Drawing for the job (mm, zero at the part's lowest x, y, z). A direction names the side the tool comes from. Give positions to 0.01 mm unless a question says otherwise; leave off trailing zeros. Order: outer loops, then holes, each group sorted by start corner. A loop starts at its lowest first (then second) coordinate and runs counter-clockwise, first axis right, second up. Notation, with made-up numbers: (-6.5, 76) - (31.5, 76) arc R29 cw to (31.5, 104) - close; hole circle Ø4 at (49, 68.25). An arc over 180 degrees is marked (long way). Use CSV: the item, a comma, the result in double quotes. Start each with the question number.
(1) Band-saw the part on B-B, the plane y = 8.75. Give the cut face in (x, z).
(2) Tool access for the marked faces 1, 2 and 3: list every direction of +Z, -Z, +X, -X, +Y, -Y with a clear straight run to the whole face (end or side of a thin tool).
(3) Pull direction X, two halves, no side cores. Call the marked faces 4, 5 and 6: +X half, -X half, draft (parallel to the pull), parting line (faces both ways), or undercut.
(4) Drop flat-ended pins along their axis: pin 1 Ø24 at (x, z) = (36, 52.5) entering from -Y; pin 2 Ø3 at (y, z) = (20.5, 39) entering from +X; pin 3 Ø2 at (x, z) = (44.5, 67) entering from +Y; pin 4 Ø10 at (y, z) = (3.5, 12.5) entering from +X. Give the stop position or say it passes through.
(5) Probe L1, parallel to Z at x = 50, y = 7; L2, parallel to X at y = 8, z = 59; L3, parallel to Z at x = 50, y = 12.75. List the from-to ranges inside material, lowest first.
(6) Band-saw the part on C-C, the plane z = 50. Give the cut face in (x, y).
(7) Band-saw the part on A-A, the plane x = 50. Give the cut face in (y, z), then the cut area to 3 significant figures.
(8) Band-saw the part on D-D, the plane z = 65. Give the cut face in (x, y).
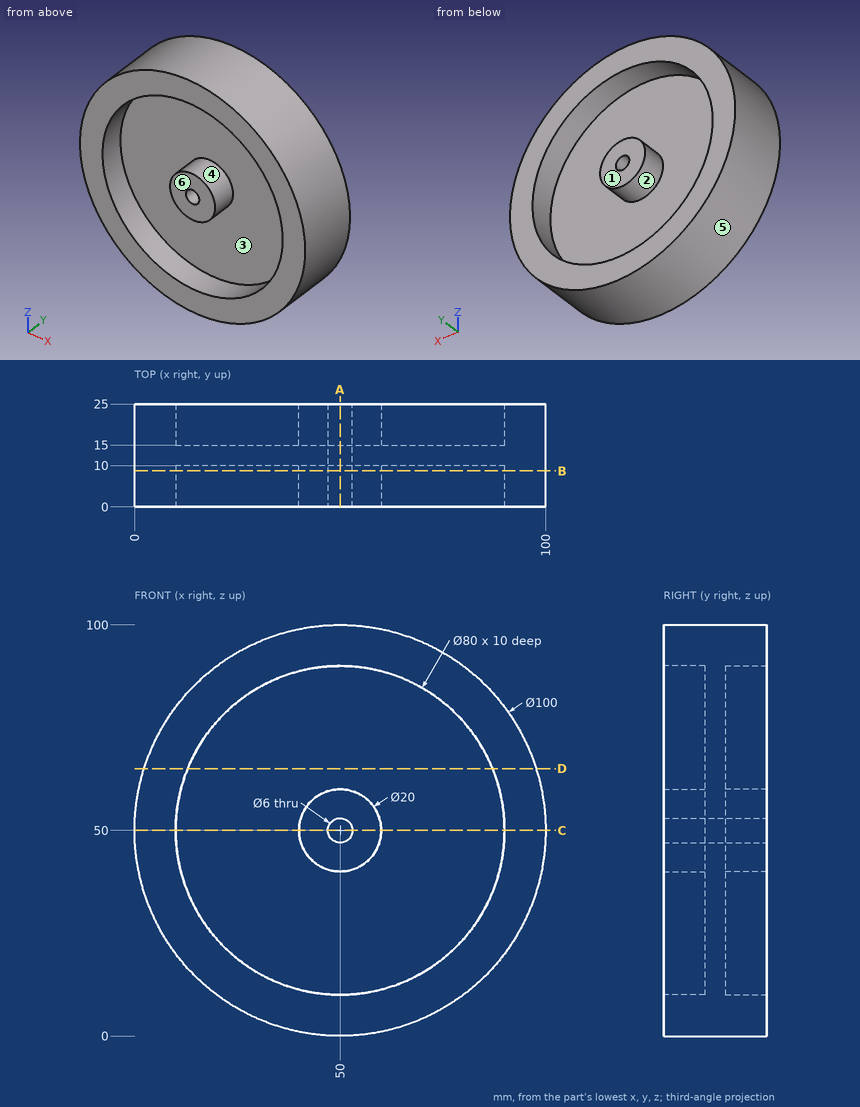
Answer block:
1,outline,"circle Ø100 at (50, 50); circle Ø20 at (50, 50); hole circle Ø80 at (50, 50); hole circle Ø6 at (50, 50)"
2,face 1,"+Z, -Z, +X, -X, +Y"
2,face 2,"+Y"
2,face 3,"-Y"
3,face 4,"undercut"
3,face 5,"parting line"
3,face 6,"draft"
4,pin 1,"stops at y = 0"
4,pin 2,"stops at x = 99.09"
4,pin 3,"stops at y = 15"
4,pin 4,"stops at x = 88"
5,L1,"z = 0 to 10, 40 to 47, 53 to 60, 90 to 100"
5,L2,"x = 0.82 to 11.03, 45.64 to 54.36, 88.97 to 99.18"
5,L3,"z = 0 to 47, 53 to 100"
6,outline,"(0, 0) - (10, 0) - (10, 10) - (40, 10) - (40, 0) - (47, 0) - (47, 25) - (40, 25) - (40, 15) - (10, 15) - (10, 25) - (0, 25) - close; (53, 0) - (60, 0) - (60, 10) - (90, 10) - (90, 0) - (100, 0) - (100, 25) - (90, 25) - (90, 15) - (60, 15) - (60, 25) - (53, 25) - close"
7,outline,"(0, 0) - (25, 0) - (25, 10) - (15, 10) - (15, 40) - (25, 40) - (25, 47) - (0, 47) - (0, 40) - (10, 40) - (10, 10) - (0, 10) - close; (0, 53) - (25, 53) - (25, 60) - (15, 60) - (15, 90) - (25, 90) - (25, 100) - (0, 100) - (0, 90) - (10, 90) - (10, 60) - (0, 60) - close"
7,area,"1,150 mm2"
8,outline,"(2.3, 0) - (12.92, 0) - (12.92, 10) - (87.08, 10) - (87.08, 0) - (97.7, 0) - (97.7, 25) - (87.08, 25) - (87.08, 15) - (12.92, 15) - (12.92, 25) - (2.3, 25) - close"
